from build123d import *

# Parameters (mm, degrees)
SKETCH_R        = 5
PAD_DEPTH       = 20
SKETCH001_R     = 3.375
POCKET_DEPTH    = 17
SKETCH002_R     = 1.5
POCKET001_DEPTH = 20.001


with BuildPart() as part:
    # Sketch → Pad (new body)
    with BuildSketch(Plane.XY):
        Circle(SKETCH_R)
    extrude(amount=PAD_DEPTH)

    # Sketch001 → Pocket (cut)
    with BuildSketch(Plane(origin=(0, 0, 0), x_dir=(1, 0, 0), z_dir=(0, 0, -1))):
        Circle(SKETCH001_R)
    extrude(amount=-POCKET_DEPTH, mode=Mode.SUBTRACT)

    # Sketch002 → Pocket001 (cut, through all)
    with BuildSketch(Plane.XY.offset(20)):
        Circle(SKETCH002_R)
    extrude(amount=-POCKET001_DEPTH, mode=Mode.SUBTRACT)


solid = part.part
Read the model definition and answer for the solid it produces. Units are mm, in the model's axes. Round coordinates to 2 decimals unless told otherwise and drop trailing zeros. Loops run counter-clockwise (first coordinate to the right, second up) from the corner with the lowest first, then second, coordinate; pieces in that order, holes last.
Q1. Determine the mould class of faces 1 (the face through (-0.7, 3.3, 8.4)), 2 (the face through (-1.2, 1.2, 20)), 3 (the face through (1.5, 0.7, 17)), 4 (the face through (-1.08, -4.88, 9.86)) for opening direction Y: released by +Y, released by -Y, zero draft, split by the parting line, or undercut.
Q2. Section C-C on z = 13.5 is taken. Write down the section's boundary in (x, y) (3 decimals), and give its area (3 significant figures).
Q3. Consider probe 1 along Y at (x, z) = (0, 3.75) (3 decimals); probe 2 along Y at (x, z) = (0, 18.9); probe 3 along Z at (x, y) = (-0.25, -2). Determine where each line is inside the solid, lowest interval first.
Q4. Each of these flat-tipped pins is pushed along its axis until it touches: pin 1 (4 mm diameter, centred on x = -4, y = 1.5, fed in from -Z); pin 2 (1.5 mm diameter, centred on x = 0, y = -2.5, fed in from -Z). Where does it stop, or does it pass through?
Q5. Section A-A on y = 0 is taken. Write down the section's boundary in (x, z) (3 decimals), and give its area (4 significant figures).
Q6. Section D-D on y = 2.75 is taken. Write down the section's boundary in (x, z), and give its area (3 significant figures).
Output:
1. face 1: undercut
1. face 2: zero draft
1. face 3: undercut
1. face 4: split by the parting line
2. outline: circle Ø10 at (0, 0); hole circle Ø6.75 at (0, 0)
2. area: 42.8 mm2
3. probe 1: y = -5 to -3.375, 3.375 to 5
3. probe 2: y = -5 to -1.5, 1.5 to 5
3. probe 3: z = 17 to 20
4. pin 1: stops at z = 0
4. pin 2: stops at z = 17
5. outline: (-5, 0) - (-3.375, 0) - (-3.375, 17) - (-1.5, 17) - (-1.5, 20) - (-5, 20) - close; (1.5, 17) - (3.375, 17) - (3.375, 0) - (5, 0) - (5, 20) - (1.5, 20) - close
5. area: 76.25 mm2
6. outline: (-4.18, 0) - (-1.96, 0) - (-1.96, 17) - (1.96, 17) - (1.96, 0) - (4.18, 0) - (4.18, 20) - (-4.18, 20) - close
6. area: 101 mm2
